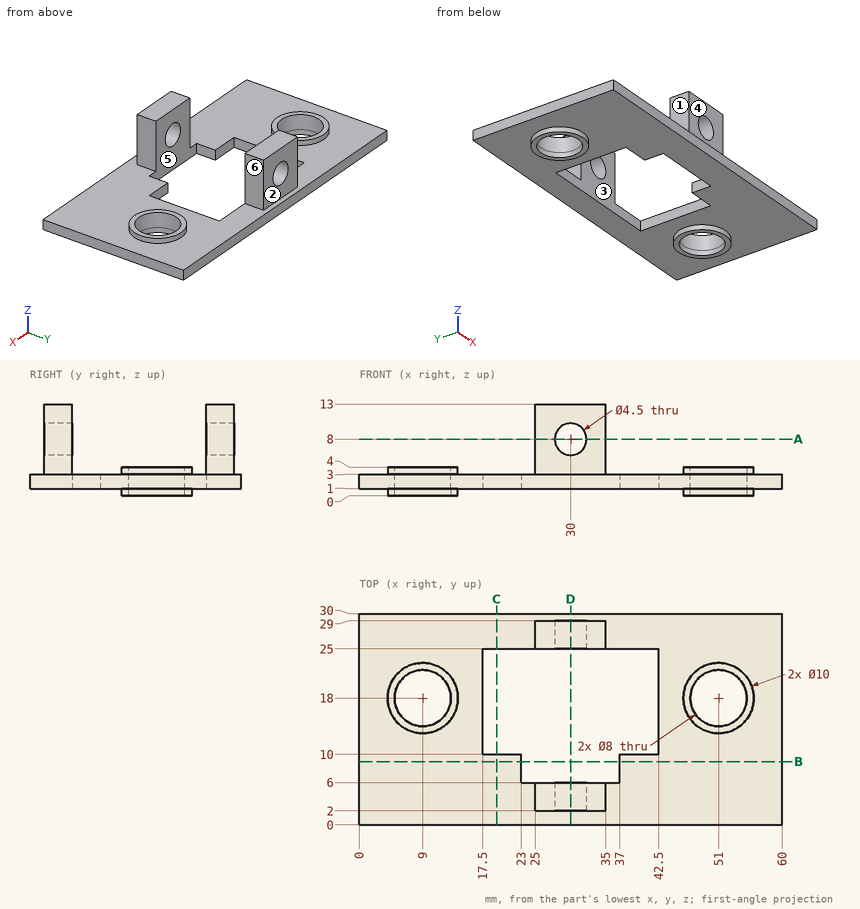
Drawing for the job (mm, zero at the part's lowest x, y, z). A direction names the side the tool comes from. Round coordinates to 2 decimals unless told otherwise and drop trailing zeros. Write each loop counter-clockwise with the first axis right and the second up, starting at its lowest first coordinate (ties: lowest second). Pieces come first, ordered by that corner, then holes. Notation, with made-up numbers: M 41,17.25 L 72,17.25 A28 cw 72,55.25 Z; hole C 83.25,18 d1. An arc over 180 degrees is marked long. Answer in a Markdown table with one row per item.
1. Which spindle directions (+Z, -Z, +X, -X, +Y, -Y) get a long thin tool onto all of the face, cutting with end or side? Do the marked faces 4, 5 and 6. Say none if no direction does.
Geometry check:
| item | result |
|---|---|
| face 4 | +Z, +X, -X, -Y |
| face 5 | +Z, -Z |
| face 6 | +Z, +X, +Y, -Y |
2. Flat gauge pins, fed straight in: P1, Ø1.2, axis at y = 28, z = 8, coming from the -X side; P2, Ø1.2, axis at y = 26.5, z = 7, coming from the +X side; P3, Ø5, axis at x = 27.5, z = 6, coming from the +Y side; P4, Ø3, axis at x = 20, y = 14.5, coming from the -Z side. Where does each tip first touch, or does it go through?
Geometry check:
| item | result |
|---|---|
| P1 | x = 25 |
| P2 | x = 35 |
| P3 | y = 29 |
| P4 | through |
3. Saw through at A-A (z = 8). List the corners of the cut face in (x, y).
Geometry check:
| item | result |
|---|---|
| outline | M 25,2 L 27.75,2 L 27.75,6 L 25,6 Z; M 25,25 L 27.75,25 L 27.75,29 L 25,29 Z; M 32.25,2 L 35,2 L 35,6 L 32.25,6 Z; M 32.25,25 L 35,25 L 35,29 L 32.25,29 Z |
4. Probe L1, parallel to Y at x = 51, z = 2.5; L2, parallel to Y at x = 9, z = 0.4; L3, parallel to Z at x = 54, y = 24.75. List the from-to ranges inside material, lowest first. Write a range as [from, to].
Geometry check:
| item | result |
|---|---|
| L1 | [0, 14], [22, 30] |
| L2 | [13, 14], [22, 23] |
| L3 | [1, 3] |
5. Saw through at B-B (y = 9). List the corners of the cut face in (x, z), and give its area (3 significant figures).
Geometry check:
| item | result |
|---|---|
| outline | M 0,1 L 23,1 L 23,3 L 0,3 Z; M 37,1 L 60,1 L 60,3 L 37,3 Z |
| area | 92.0 mm2 |
6. Saw through at C-C (x = 19.5). List the corners of the cut face in (y, z).
Geometry check:
| item | result |
|---|---|
| outline | M 0,1 L 10,1 L 10,3 L 0,3 Z; M 25,1 L 30,1 L 30,3 L 25,3 Z |
7. Mould opens along X. For the marked faces 1, 2 and 3 say: +X half, -X half, draft (parallel to the pull), parting line (faces both ways), or undercut.
Geometry check:
| item | result |
|---|---|
| face 1 | -X half |
| face 2 | draft |
| face 3 | undercut |
8. Saw through at D-D (x = 30). List the corners of the cut face in (y, z), and give its area (3 significant figures).
Geometry check:
| item | result |
|---|---|
| outline | M 0,1 L 6,1 L 6,5.75 L 2,5.75 L 2,3 L 0,3 Z; M 2,10.25 L 6,10.25 L 6,13 L 2,13 Z; M 25,1 L 30,1 L 30,3 L 29,3 L 29,5.75 L 25,5.75 Z; M 25,10.25 L 29,10.25 L 29,13 L 25,13 Z |
| area | 66.0 mm2 |
